from build123d import *

# Parameters (mm, degrees)
F1_R = 13.49375
F3_R = 11.1125


with BuildPart() as f2:
    # F2: sweep along a path in F0
    with BuildLine(Plane.XZ) as f2_path:
        Line((46.0375, 46.0375), (27.051, 46.0375))
        ThreePointArc((27.051, 46.0375), (7.9230544621, 38.1144455379), (0, 18.9865))
        Line((0, 18.9865), (0, 0))
    # F1 (on Top) → F2 (sweep)
    with BuildSketch(Plane.XY):
        with Locations((13.49375, 0)):
            Circle(F1_R)
    sweep(path=f2_path.line)

    # F4: sweep along a path in F0
    with BuildLine(Plane.XZ) as f4_path:
        Line((46.0375, 46.0375), (27.051, 46.0375))
        ThreePointArc((27.051, 46.0375), (7.9230544621, 38.1144455379), (0, 18.9865))
        Line((0, 18.9865), (0, 0))
    # F3 (on face) → F4 (sweep, cut)
    with BuildSketch(Plane(origin=(0, 0, 0), x_dir=(1, 0, 0), z_dir=(0, 0, -1))):
        with Locations((13.49375, 0)):
            Circle(F3_R)
    sweep(path=f4_path.line, mode=Mode.SUBTRACT)


solid = f2.part
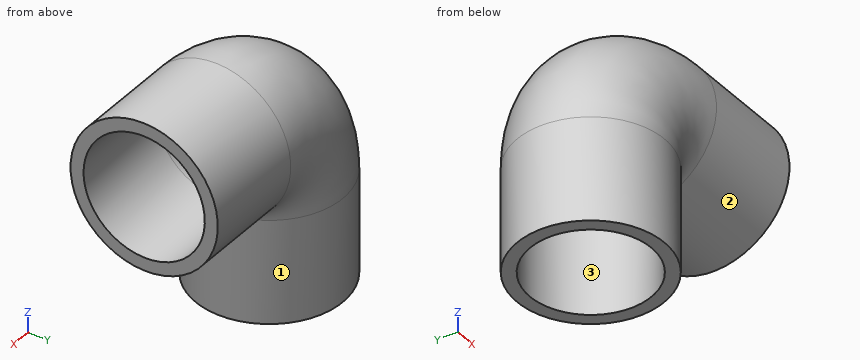
Verification items for the finished model (mm, model axes). Face numbers are marked on the shaded views. Round coordinates to 2 decimals unless told otherwise and drop trailing zeros. Write each loop counter-clockwise with the first axis right and the second up, starting at its lowest first coordinate (ties: lowest second). Pieces come first, ordered by that corner, then holes.
(1) Section check A-A (y = 0). Enter the section's corners in (x, z).
Returned:
outline: (0, 0) - (2.38, 0) - (2.38, 18.99) arc R24.67 cw to (27.05, 43.66) - (46.04, 43.66) - (46.04, 46.04) - (27.05, 46.04) arc R27.05 ccw to (0, 18.99) - close; (24.61, 0) - (26.99, 0) - (26.99, 18.99) arc R0.06 cw to (27.05, 19.05) - (46.04, 19.05) - (46.04, 21.43) - (27.05, 21.43) arc R2.44 ccw to (24.61, 18.99) - close
(2) Depth check by flat-ended pin: pin 1 Ø5 at (y, z) = (-6.5, 15.5) entering from +X; pin 2 Ø6 at (x, y) = (18.5, 1.5) entering from +Z; pin 3 Ø12 at (x, y) = (18.5, -8.5) entering from +Z. Enter the tip coordinate at first touch or a pass-through.
Returned:
pin 1: stops at x = 26.38
pin 2: stops at z = 45.42
pin 3: stops at z = 45.06
(3) Mould release check, pull along X, two halves, no side actions. Record for the marked faces 1, 2 and 3: pulls with the +X half, pulls with the -X half, needs draft (parallel to the pull), parting line crosses it, or undercut.
Returned:
face 1: parting line crosses it
face 2: needs draft
face 3: undercut
(4) Material ranges on line 1 (Z direction, x = 31.25, y = 0); line 2 (X direction, y = 2, z = 7); line 3 (Z direction, x = 31.5, y = 1.5), recorded low to high.
Returned:
line 1: z = 19.05 to 21.43, 43.66 to 46.04
line 2: x = 0.15 to 2.56, 24.42 to 26.84
line 3: z = 19.13 to 21.53, 43.55 to 45.95
(5) Section check C-C (y = -7.75). Enter the section's corners in (x, z).
Returned:
outline: (2.45, 0) - (5.53, 0) - (5.53, 18.99) arc R21.52 cw to (27.05, 40.51) - (46.04, 40.51) - (46.04, 43.59) - (27.05, 43.59) arc R24.6 ccw to (2.45, 18.99) - close; (21.46, 0) - (24.54, 0) - (24.54, 18.99) arc R2.51 cw to (27.05, 21.5) - (46.04, 21.5) - (46.04, 24.58) - (27.05, 24.58) arc R5.59 ccw to (21.46, 18.99) - close
(6) Section check B-B (z = 4). Enter the section's corners in (x, y) (1 decimal), plus the area to 3 significant figures.
Returned:
outline: circle Ø27 at (13.5, 0); hole circle Ø22.2 at (13.5, 0)
area: 184 mm2
